from build123d import *

# Parameters (mm, degrees)
SKETCH_1_W      = 130
SKETCH_1_H      = 24.8
EXTRUDE_1_DEPTH = 5


with BuildPart() as part:
    # 草图1 → 凸台-拉伸1 (new body)
    with BuildSketch(Plane.XY):
        Polygon((-130, -7.5), (-130, 0), (-130, 24.8), (-130, 32.5), (-150, 32.5), (-150, -7.5), align=None)
        with Locations((-65, 12.4)):
            Rectangle(SKETCH_1_W, SKETCH_1_H)
    extrude(amount=EXTRUDE_1_DEPTH)


solid = part.part
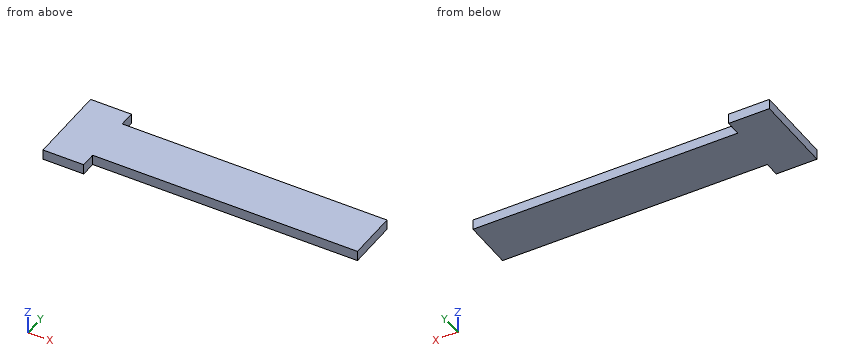
Can you work these out from the model? Positions are in its coordinate system, mm. Give positions to 0.01 mm unless a question says otherwise; leave off trailing zeros. Loops run counter-clockwise (first coordinate to the right, second up) from the corner with the lowest first, then second, coordinate; pieces in that order, holes last. Notation, with made-up numbers: (62, -18.5) -> (91, -18.5) arc R5 ccw to (91, -13.5) -> close; hole circle Ø5 at (-26.75, 5). An arc over 180 degrees is marked (long way). Use one line per item in the form item = value.
1) If we section it at C-C (y = 26.5): Please give me the cut outline in (x, z).
Answers:
outline = (-150, 0) -> (-130, 0) -> (-130, 5) -> (-150, 5) -> close
2) If we section it at A-A (z = 2.95): Please give me the cut outline in (x, y), plus the area to 3 significant figures.
Answers:
outline = (-150, -7.5) -> (-130, -7.5) -> (-130, 0) -> (0, 0) -> (0, 24.8) -> (-130, 24.8) -> (-130, 32.5) -> (-150, 32.5) -> close
area = 4,020 mm²
3) If we section it at B-B (x = -62): Please give me the cut outline in (y, z).
Answers:
outline = (0, 0) -> (24.8, 0) -> (24.8, 5) -> (0, 5) -> close
4) Will these pins go through, and if not, where does the flat tip stop? pin 1 (2.5 mm diameter, centred on x = -80.5, z = 2, fed in from -Y); pin 2 (1.5 mm diameter, centred on x = -25.5, z = 1.5, fed in from +Y).
Answers:
pin_1 = 0
pin_2 = 24.8
5) I need wall thicknesses on line 1 along Y through (x, z) = (-15, 3.95). Which ranges of the line are inside material? Lowest first, please.
Answers:
line_1 = 0 to 24.8
